Read the model definition and answer for the solid it produces. Units are mm, in the model's axes. Face numbers are marked on the shaded views. A direction names the side the tool comes from. Round coordinates to 2 decimals unless told otherwise and drop trailing zeros. Order: outer loops, then holes, each group sorted by start corner. A loop starts at its lowest first (then second) coordinate and runs counter-clockwise, first axis right, second up. Notation, with made-up numbers: (-33, 27.25) -> (17, 27.25) arc R24 cw to (17, 37.25) -> close; hole circle Ø2 at (-27, -11). An arc over 180 degrees is marked (long way). Use a Markdown table: item, result. Add a question column.
1. For the marked faces 1, 2, 3, 4 and 5, determine the directions among +Z, -Z, +X, -X, +Y, -Y from which every point of the face is accessible in a straight line to the end or side of a thin tool.
2. Consider L1, parallel to X at y = -16, z = 1; L2, parallel to Y at x = 40.5, z = 30.5; L3, parallel to Z at x = 14.5, y = -31. Determine where each line is inside the solid, lowest interval first. Write a range as [from, to].
3. Section C-C, the plane x = 40.5 is taken. Give the vertices of the cut face in (y, z), then the cut area to 3 significant figures.
4. Given pin 1 (6 mm diameter, centred on x = 15.5, z = 9, fed in from +Y); pin 2 (0.8 mm diameter, centred on x = 34.5, z = 16.5, fed in from +Y); pin 3 (5 mm diameter, centred on x = 24, y = -13, fed in from +Z); pin 4 (5 mm diameter, centred on y = -19, z = 16.5, fed in from +X), each flat-ended and moving along its own axis, determine where each tip first touches the part or whether it passes through.
5. Section D-D, the plane z = 26.5 is taken. Give the vertices of the cut face in (x, y).
6. Section B-B, the plane z = 5 is taken. Give the vertices of the cut face in (x, y), then the cut area to 3 significant figures.
7. The mould has two halves that part along X. Classify the marked faces 6, 7 and 8: +X half, -X half, draft (parallel to the pull), parting line (faces both ways), or undercut.
8. Section A-A, the plane x = 32 is taken. Give the vertices of the cut face in (y, z), then the cut area to 3 significant figures.
```python
from build123d import *

# Parameters (mm, degrees)
F0_W     = 63.5
F0_H     = 38.1
F1_DEPTH = 6.35
F2_W     = 0.7357047051
F2_H     = 2.4810375154
F3_DEPTH = 25.4
F4_W     = 7.62
F4_H     = 7.62
F5_DEPTH = 6.35


with BuildPart() as f1:
    # F0 (on Top) → F1 (new body)
    with BuildSketch(Plane.XY):
        with Locations((31.75, -19.05)):
            Rectangle(F0_W, F0_H)
    extrude(amount=F1_DEPTH)

    # F2 (on face) → F3 (join)
    with BuildSketch(Plane.XY.offset(6.35)):
        with Locations((31.3821476474, -17.8094812423)):
            Rectangle(F2_W, F2_H)
        Polygon((33.1730134785, -16.5689624846), (31.75, -16.5689624846), (31.75, -19.05), (44.3069849849, -19.05), (44.3069849849, -14.2875), (34.7819849849, -14.2875), (34.7819849849, -17.6186021417), (33.1730134785, -17.6186021417), align=None)
        with Locations((31.3821476474, -20.2905187577)):
            Rectangle(F2_W, F2_H)
        Polygon((44.3069849849, -19.05), (31.75, -19.05), (31.75, -21.5310375154), (33.1730134785, -21.5310375154), (33.1730134785, -20.4813978583), (34.7819849849, -20.4813978583), (34.7819849849, -23.8125), (44.3069849849, -23.8125), align=None)
    extrude(amount=F3_DEPTH)

    # F4 (on face) → F5 (cut)
    with BuildSketch(Plane(origin=(0, 0, 0), x_dir=(1, 0, 0), z_dir=(0, 0, -1))):
        with Locations((27.94, 15.24)):
            Rectangle(F4_W, F4_H)
        with Locations((35.56, 15.24)):
            Rectangle(F4_W, F4_H)
        with Locations((35.56, 22.86)):
            Rectangle(F4_W, F4_H)
        with Locations((27.94, 22.86)):
            Rectangle(F4_W, F4_H)
    extrude(amount=-F5_DEPTH, mode=Mode.SUBTRACT)


solid = f1.part
```
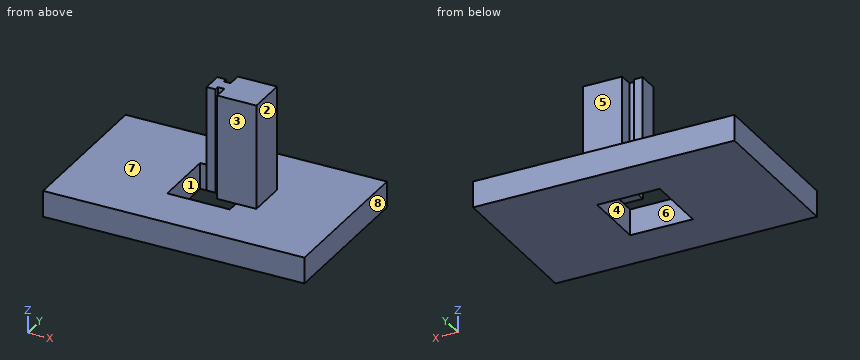
Verdict:
| question | item | result |
|---|---|---|
| 1 | face 1 | +Z, -Z |
| 1 | face 2 | +Z, +X, +Y, -Y |
| 1 | face 3 | +Z, +X, -X, -Y |
| 1 | face 4 | -Z |
| 1 | face 5 | +Z, +X, -X, +Y |
| 2 | L1 | x = [0, 24.13], [39.37, 63.5] |
| 2 | L2 | y = [-23.81, -14.29] |
| 2 | L3 | z = [0, 6.35] |
| 3 | outline | (-38.1, 0) -> (0, 0) -> (0, 6.35) -> (-14.29, 6.35) -> (-14.29, 31.75) -> (-23.81, 31.75) -> (-23.81, 6.35) -> (-38.1, 6.35) -> close |
| 3 | area | 484 mm2 |
| 4 | pin 1 | stops at y = 0 |
| 4 | pin 2 | stops at y = -14.29 |
| 4 | pin 3 | stops at z = 6.35 |
| 4 | pin 4 | stops at x = 44.31 |
| 5 | outline | (31.01, -21.53) -> (33.17, -21.53) -> (33.17, -20.48) -> (34.78, -20.48) -> (34.78, -23.81) -> (44.31, -23.81) -> (44.31, -14.29) -> (34.78, -14.29) -> (34.78, -17.62) -> (33.17, -17.62) -> (33.17, -16.57) -> (31.01, -16.57) -> close |
| 6 | outline | (0, -38.1) -> (63.5, -38.1) -> (63.5, 0) -> (0, 0) -> close; hole (24.13, -26.67) -> (39.37, -26.67) -> (39.37, -11.43) -> (24.13, -11.43) -> close |
| 6 | area | 2,190 mm2 |
| 7 | face 6 | undercut |
| 7 | face 7 | draft |
| 7 | face 8 | +X half |
| 8 | outline | (-38.1, 0) -> (-26.67, 0) -> (-26.67, 6.35) -> (-38.1, 6.35) -> close; (-21.53, 6.35) -> (-16.57, 6.35) -> (-16.57, 31.75) -> (-21.53, 31.75) -> close; (-11.43, 0) -> (0, 0) -> (0, 6.35) -> (-11.43, 6.35) -> close |
| 8 | area | 271 mm2 |
